Input: dimensioned drawing with shaded views. Units: mm. Origin: part minimum x, y, z. A direction names the side the tool comes from. Give positions to 0.01 mm unless a question says otherwise; leave off trailing zeros. Write each loop counter-clockwise with the first axis right and the second up, starting at its lowest first coordinate (ties: lowest second). Pieces come first, ordered by that corner, then holes. Notation, with made-up numbers: (34.5, 1.25) -> (54.5, 1.25) arc R23 ccw to (54.5, 20.25) -> close; hole circle Ø8 at (-5, 2.5). An arc over 180 degrees is marked (long way). Answer as a JSON object with one key per item and string values.
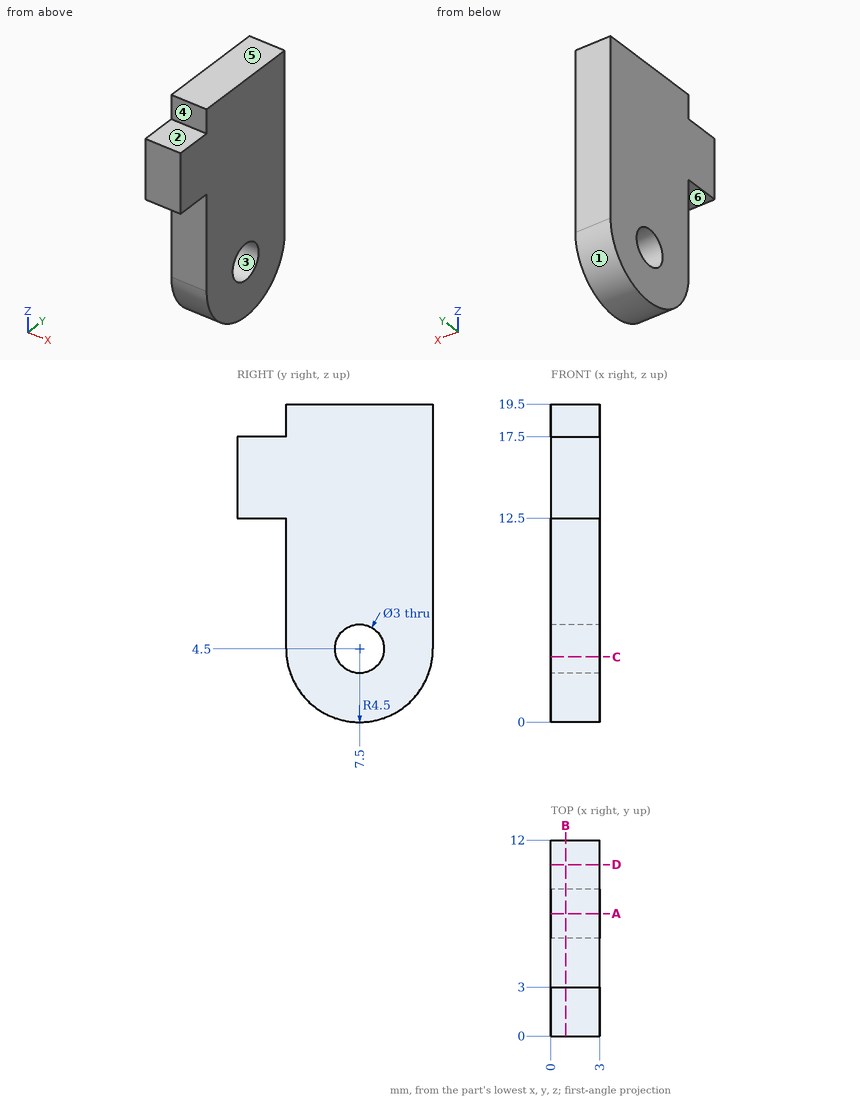
Q1. Cut plane D-D (y = 10.5). Return the cut outline in (x, z).
Values:
{"outline": "(0, 1.15) -> (3, 1.15) -> (3, 19.5) -> (0, 19.5) -> close"}
Q2. Material intervals for L1, parallel to Y at x = 1.75, z = 4.5; L2, parallel to Z at x = 1.7, y = 2; L3, parallel to Y at x = 2.05, z = 18.25, sorted ascending. Write a range as from..to.
Values:
{"L1": "3..6, 9..12", "L2": "12.5..17.5", "L3": "3..12"}
Q3. Cut plane A-A (y = 7.5). Return the cut outline in (x, z), and give its area (3 significant figures).
Values:
{"outline": "(0, 0) -> (3, 0) -> (3, 3) -> (0, 3) -> close; (0, 6) -> (3, 6) -> (3, 19.5) -> (0, 19.5) -> close", "area": "49.5 mm²"}
Q4. Cut plane B-B (x = 0.9). Return the cut outline in (y, z).
Values:
{"outline": "(0, 12.5) -> (3, 12.5) -> (3, 4.5) arc R4.5 ccw to (12, 4.5) -> (12, 19.5) -> (3, 19.5) -> (3, 17.5) -> (0, 17.5) -> close; hole circle Ø3 at (7.5, 4.5)"}
Q5. Set-up query: the marked faces 4, 5 and 6. Return all of +Z, -Z, +X, -X, +Y, -Y with unobstructed straight access to the full face (end or side cutting, diameter ignored); none if empty.
Values:
{"face 4": "+Z, +X, -X, -Y", "face 5": "+Z, +X, -X, +Y, -Y", "face 6": "-Z, +X, -X, -Y"}
Q6. First-contact query: P1, Ø0.9, axis at x = 2, y = 2, coming from the +Z side; P2, Ø2.5, axis at y = 7.5, z = 4.5, coming from the -X side; P3, Ø1.6, axis at x = 1, z = 18.5, coming from the -Y side. Flat tips, straight axial feed; report the tip coordinate or a pass-through.
Values:
{"P1": "z = 17.5", "P2": "through", "P3": "y = 3"}
Q7. Mould query, pull axis Y, two halves, no side actions, for the marked faces 1, 2 and 3. Classes: pulls with the +Y half, pulls with the -Y half, needs draft (parallel to the pull), parting line crosses it, or undercut.
Values:
{"face 1": "parting line crosses it", "face 2": "needs draft", "face 3": "undercut"}
Q8. Cut plane C-C (z = 4). Return the cut outline in (x, y).
Values:
{"outline": "(0, 3.03) -> (3, 3.03) -> (3, 6.09) -> (0, 6.09) -> close; (0, 8.91) -> (3, 8.91) -> (3, 11.97) -> (0, 11.97) -> close"}
